from build123d import *

# Parameters (mm, degrees)
SKETCH1_W           = 98
SKETCH1_H           = 60
BOSS_EXTRUDE1_DEPTH = 1.6
SKETCH2_W           = 97
SKETCH2_H           = 39.5
BOSS_EXTRUDE2_DEPTH = 9.9
SKETCH4_R           = 1.5
CUT_EXTRUDE1_DEPTH  = 1.6
SKETCH5_R           = 0.5
CUT_EXTRUDE2_DEPTH  = 1.6
SKETCH6_W           = 40.313195669
SKETCH6_H           = 1.990775095
BOSS_EXTRUDE3_DEPTH = 6
SKETCH3_W           = 76
SKETCH3_H           = 26
CUT_EXTRUDE3_DEPTH  = 0.254


with BuildPart() as part:
    # Sketch1 → Boss-Extrude1 (new body)
    with BuildSketch(Plane(origin=(0, 0, 0), x_dir=(1, 0, 0), z_dir=(0, 1, 0))):
        with Locations((-23.16287695, -6.675720991)):
            Rectangle(SKETCH1_W, SKETCH1_H)
    extrude(amount=BOSS_EXTRUDE1_DEPTH)

    # Sketch2 → Boss-Extrude2 (add)
    with BuildSketch(Plane(origin=(0, 1.6, 0), x_dir=(1, 0, 0), z_dir=(0, 1, 0))):
        with Locations((-23.16287695, -6.675720991)):
            Rectangle(SKETCH2_W, SKETCH2_H)
    extrude(amount=BOSS_EXTRUDE2_DEPTH)

    # Sketch4 → Cut-Extrude1 (cut)
    with BuildSketch(Plane(origin=(0, 1.6, 0), x_dir=(1, 0, 0), z_dir=(0, 1, 0))):
        with Locations((-69.16287695, -34.675720991)):
            Circle(SKETCH4_R)
        with Locations((23.83712305, -34.675720991)):
            Circle(SKETCH4_R)
        with Locations((-69.16287695, 20.324279009)):
            Circle(SKETCH4_R)
        with Locations((23.83712305, 20.324279009)):
            Circle(SKETCH4_R)
    extrude(amount=-CUT_EXTRUDE1_DEPTH, mode=Mode.SUBTRACT)

    # Sketch5 → Cut-Extrude2 (cut)
    with BuildSketch(Plane(origin=(0, 1.6, 0), x_dir=(1, 0, 0), z_dir=(0, 1, 0))):
        with Locations((15.73712305, -33.575720991)):
            Circle(SKETCH5_R)
        with Locations((13.19712305, -33.575720991)):
            Circle(SKETCH5_R)
        with Locations((10.65712305, -33.575720991)):
            Circle(SKETCH5_R)
        with Locations((8.11712305, -33.575720991)):
            Circle(SKETCH5_R)
        with Locations((5.57712305, -33.575720991)):
            Circle(SKETCH5_R)
        with Locations((3.03712305, -33.575720991)):
            Circle(SKETCH5_R)
        with Locations((0.49712305, -33.575720991)):
            Circle(SKETCH5_R)
        with Locations((-2.04287695, -33.575720991)):
            Circle(SKETCH5_R)
        with Locations((-4.58287695, -33.575720991)):
            Circle(SKETCH5_R)
        with Locations((-7.12287695, -33.575720991)):
            Circle(SKETCH5_R)
        with Locations((-9.66287695, -33.575720991)):
            Circle(SKETCH5_R)
        with Locations((-12.20287695, -33.575720991)):
            Circle(SKETCH5_R)
        with Locations((-14.74287695, -33.575720991)):
            Circle(SKETCH5_R)
        with Locations((-17.28287695, -33.575720991)):
            Circle(SKETCH5_R)
        with Locations((-19.82287695, -33.575720991)):
            Circle(SKETCH5_R)
        with Locations((-22.36287695, -33.575720991)):
            Circle(SKETCH5_R)
    extrude(amount=-CUT_EXTRUDE2_DEPTH, mode=Mode.SUBTRACT)

    # Sketch6 → Boss-Extrude3 (add)
    with BuildSketch(Plane.XZ):
        with Locations((-3.241605768, 33.478976188)):
            Rectangle(SKETCH6_W, SKETCH6_H)
    extrude(amount=BOSS_EXTRUDE3_DEPTH)

    # Sketch3 → Cut-Extrude3 (cut)
    with BuildSketch(Plane(origin=(0, 11.5, 0), x_dir=(1, 0, 0), z_dir=(0, 1, 0))):
        with Locations((-23.766549937, -6.888251248)):
            Rectangle(SKETCH3_W, SKETCH3_H)
    extrude(amount=-CUT_EXTRUDE3_DEPTH, mode=Mode.SUBTRACT)


solid = part.part
Can you work these out from the model? Positions are in its coordinate system, mm. A direction names the side the tool comes from. Coordinates: 2 decimals unless noted, no trailing zeros. Write each loop counter-clockwise with the first axis right and the second up, starting at its lowest first coordinate (ties: lowest second). Pieces come first, ordered by that corner, then holes. Notation, with made-up numbers: (42.25, 25) -> (100.25, 25) arc R32 ccw to (100.25, 59) -> close; hole circle Ø10 at (22, 39). An arc over 180 degrees is marked (long way). Write item = value, one per line.
(1) On a 3-axis mill with a long thin cutter (end or side, diameter ignored), from which of +Z, -Z, +X, -X, +Y, -Y can I reach the whole of each face in a straight line? I mean faces 5 (the face through (-71.663, 6, 7)), 6 (the face through (-24, 6, 26.426)), 7 (the face through (-4, -3, 32.484)), 8 (the face through (16.915, -3, 33)), 9 (the face through (-23.398, -3, 33)). Say none if no direction works.
Verdict:
face_5 = +Z, -Z, -X, +Y
face_6 = +Z, +X, -X, +Y
face_7 = -Z, +X, -X, -Y
face_8 = +Z, -Z, +X, -Y
face_9 = +Z, -Z, -X, -Y
(2) Thinking about a two-plate mould opening in Z: for faces 1 (the face through (-24, 0, 6)), 2 (the face through (-24, 11.246, 7)), 3 (the face through (-24, 6, -13.074)), 4 (the face through (-4, -3, 34.474)), which applies, +Z half, -Z half, draft (parallel to the pull), parting line (faces both ways), or undercut?
Verdict:
face_1 = draft
face_2 = undercut
face_3 = -Z half
face_4 = +Z half
(3) Imagine slicing it at B-B (x = -55). Please give me the cut outline in (y, z), and give its area (3 significant figures).
Verdict:
outline = (0, -23.32) -> (1.6, -23.32) -> (1.6, -13.07) -> (11.5, -13.07) -> (11.5, -6.11) -> (11.25, -6.11) -> (11.25, 19.89) -> (11.5, 19.89) -> (11.5, 26.43) -> (1.6, 26.43) -> (1.6, 36.68) -> (0, 36.68) -> close
area = 480 mm^2
(4) Imagine slicing it at C-C (y = -2.5). Please give me the cut outline in (x, z) (3 decimals), and give its area (3 significant figures).
Verdict:
outline = (-23.398, 32.484) -> (16.915, 32.484) -> (16.915, 34.474) -> (-23.398, 34.474) -> close
area = 80.3 mm^2
(5) Imagine slicing it at D-D (z = -5). Please give me the cut outline in (x, y).
Verdict:
outline = (-72.16, 0) -> (25.84, 0) -> (25.84, 1.6) -> (25.34, 1.6) -> (25.34, 11.5) -> (14.23, 11.5) -> (14.23, 11.25) -> (-61.77, 11.25) -> (-61.77, 11.5) -> (-71.66, 11.5) -> (-71.66, 1.6) -> (-72.16, 1.6) -> close
(6) Imagine slicing it at A-A (z = 23.5). Please give me the cut outline in (x, y), and give its area (3 significant figures).
Verdict:
outline = (-72.16, 0) -> (25.84, 0) -> (25.84, 1.6) -> (25.34, 1.6) -> (25.34, 11.5) -> (-71.66, 11.5) -> (-71.66, 1.6) -> (-72.16, 1.6) -> close
area = 1,120 mm^2
(7) If I drill on probe 1 along Y at (x, z) = (-63.5, 18); probe 2 along Y at (x, z) = (-12.5, 6.5); probe 3 along Z at (x, y) = (-43.5, 10), over which ranges is the centre line in solid material (lowest first)?
Verdict:
probe_1 = 0 to 11.5
probe_2 = 0 to 11.25
probe_3 = -13.07 to 26.43
(8) For pin 1 (0.5 mm diameter, centred on x = -17, z = 33.5, fed in from +Y); pin 2 (2 mm diameter, centred on y = -3, z = 34, fed in from +X) (3 decimals); pin 3 (2 mm diameter, centred on y = 8, z = -0.5, fed in from -X), each with a flat end and sliding along its axis, tell me the tip position at first contact or that it passes through.
Verdict:
pin_1 = 1.6
pin_2 = 16.915
pin_3 = -71.66
